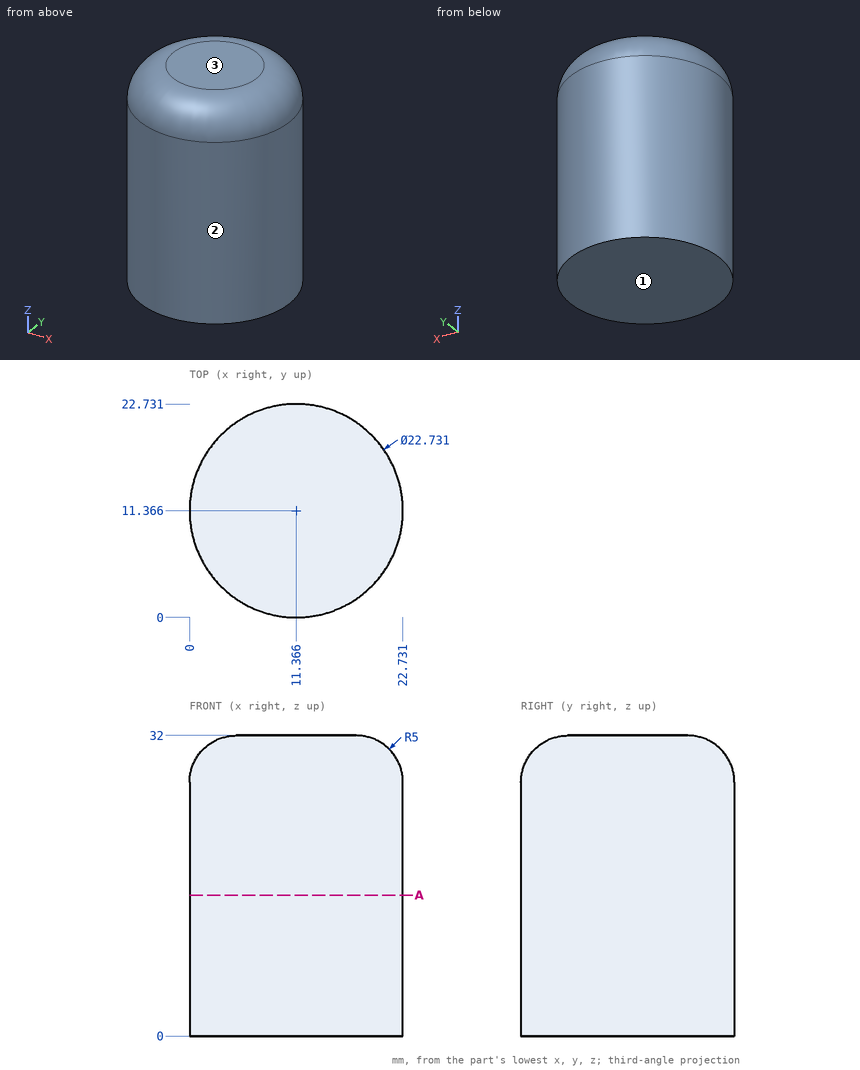
Can you work these out from the drawing? Everything is in mm from the part's minimum corner. Round coordinates to 2 decimals unless told otherwise and drop trailing zeros. Loops run counter-clockwise (first coordinate to the right, second up) from the corner with the lowest first, then second, coordinate; pieces in that order, holes last. Notation, with made-up numbers: (-9, -2) - (4, -2) arc R21 cw to (4, 3) - close; hole circle Ø7 at (28, -26.75). An arc over 180 degrees is marked (long way). Write item = value, one per line. Start each with the question number.
(1) If we section it at A-A (z = 15): Please give me the cut outline in (x, y) (1 decimal), and give its area (3 significant figures).
(2) If I drill on probe 1 along Y at (x, z) = (2.25, 26) (1 decimal); probe 2 along Z at (x, y) = (20, 9); probe 3 along X at (y, z) = (5.75, 10.5) (1 decimal), over which ranges is the centre line in solid material (lowest first)? Write a range as [from, to].
(3) For P1, Ø8, axis at x = 2.5, z = 20, coming from the +Y side; P2, Ø8, axis at y = 17, z = 8.5, coming from the +X side; P3, Ø1.5, axis at y = 7, z = 22, coming from the -X side, each with a flat end and sliding along its axis, tell me the tip position at first contact or that it passes through.
(4) If we mould it in two halves opening along Z, with no side actions, what happens to the marked faces 1, 2 and 3? For each: released by +Z, released by -Z, zero draft, split by the parting line, or undercut.
Ans:
q1.outline = circle Ø22.7 at (11.4, 11.4)
q1.area = 406 mm²
q2.probe_1 = [4.6, 18.2]
q2.probe_2 = [0, 31.28]
q2.probe_3 = [1.5, 21.2]
q3.P1 = 21.64
q3.P2 = 22.61
q3.P3 = 0.59
q4.face_1 = released by -Z
q4.face_2 = zero draft
q4.face_3 = released by +Z
